Geometry: final body of the model. Coordinates: model frame, mm. Face numbers are marked on the shaded views. A direction names the side the tool comes from. Give positions to 0.01 mm unless a question says otherwise; leave off trailing zeros. Write each loop counter-clockwise with the first axis right and the second up, starting at its lowest first coordinate (ties: lowest second). Pieces come first, ordered by that corner, then holes. Notation, with made-up numbers: (70.25, 77.5) - (111.25, 77.5) arc R35 ccw to (111.25, 110.5) - close; hole circle Ø10 at (-20.75, 17). An arc over 180 degrees is marked (long way). Use CSV: the item, a comma, the result in double quotes. Start each with the question number.
(1) Reachability of the marked faces 1 and 2 from +Z, -Z, +X, -X, +Y, -Y: full face, straight path, thin tool, end or side. Return the list, or none.
(2) Section B-B on x = 0. Output: boundary loops of the cut face in (y, z).
(3) Section D-D on x = -11. Output: boundary loops of the cut face in (y, z), and give its area (3 significant figures).
(4) First-contact query: pin 1 Ø3 at (x, z) = (-3.5, -2) entering from +Y; pin 2 Ø4 at (x, z) = (-4.5, -0.5) entering from -Y; pin 3 Ø1 at (x, y) = (5, 6) entering from +Z; pin 4 Ø4 at (y, z) = (11.5, -6) entering from -X. Flat tips, straight axial feed; report the tip coordinate or a pass-through.
(5) Draft query along X for the marked faces 3, 4 and 5. Return one class per face: released by +X, released by -X, zero draft, split by the parting line, or undercut.
(6) Line query: probe 1 along Y at (x, z) = (0, -4); probe 2 along Y at (x, z) = (0, 1.5); probe 3 along Z at (x, y) = (3.5, 13). Output: solid intervals per line, ascending. Write a range as [from, to].
(7) Section A-A on y = 1.5. Output: boundary loops of the cut face in (x, z), and give its area (3 significant figures).
(8) Section C-C on z = -11.25. Output: boundary loops of the cut face in (x, y).
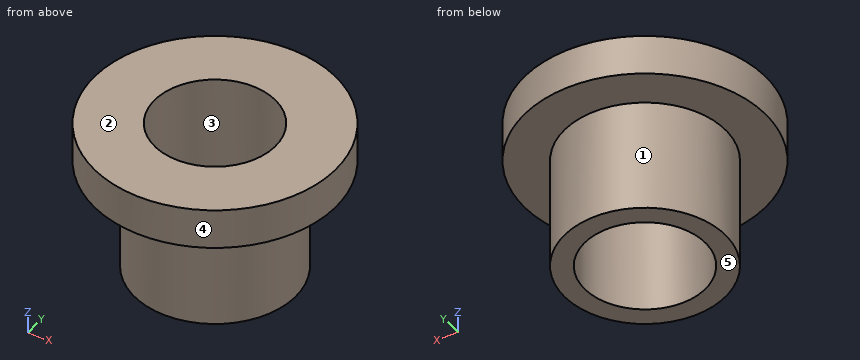
Autodesk Inventor part; units mm, degrees
ref_plane "Work Plane1" through (-46.5047, -36.7959, -17) normal (0, 0, -1) x (0, 1, 0)
ref_plane "Work Plane2" through (-46.5047, -36.7959, -14) normal (0, 0, -1) x (0, 1, 0)
ref_plane "YZ Plane" through (0, 0, 0) normal (1, 0, 0) x (0, 1, 0)
sketch "Sketch1" plane through (0, 0, 0) normal (0, 0, 1) x (1, 0, 0)
  circle A0 centre (0, 1.5) radius 10
  circle A1 centre (0, 1.5) radius 10
  circle A2 centre (0, 1.5) radius 15
  circle A3 centre (0, 1.5) radius 7.5
  point P0 (0, 0)
  dimension "d0" = 30
  dimension "d1" = 15
ref_plane "Work Plane1" through (-46.5047, -36.7959, -17) normal (0, 0, -1) x (0, 1, 0)
ref_plane "Work Plane2" through (-46.5047, -36.7959, -14) normal (0, 0, -1) x (0, 1, 0)
extrude "Extrusion1" add sketch "Sketch1" against normal up to surface (14 mm away) contours A0
sketch "Sketch2" plane through (0, 1.5, 0) normal (0, 0, 1) x (1, 0, 0)
  circle A0 centre (0, 0) radius 10
  circle A1 centre (0, 0) radius 7.5
  circle A2 centre (0, 0) radius 15
  point P0 (0, -1.5)
  dimension "d4" = 30
extrude "Extrusion2" add sketch "Sketch2" along normal blind 5 contours A0 | A2
properties part number "glide lejre bushing" material "Brass, Soft Yellow"
Check values:
1,face 1,"-Z"
1,face 2,"+Z, +X, -X, +Y, -Y"
2,outline,"(-13.5, 0) - (-8.5, 0) - (-8.5, -14) - (-6, -14) - (-6, 5) - (-13.5, 5) - close; (9, -14) - (11.5, -14) - (11.5, 0) - (16.5, 0) - (16.5, 5) - (9, 5) - close"
3,outline,"(-8.7, 0) - (11.7, 0) - (11.7, 5) - (-8.7, 5) - close"
3,area,"102 mm²"
4,pin 1,"stops at y = 11.3"
4,pin 2,"stops at y = -13.28"
4,pin 3,"passes through"
4,pin 4,"stops at x = -6"
5,face 3,"undercut"
5,face 4,"split by the parting line"
5,face 5,"zero draft"
6,probe 1,"y = [-8.5, -6], [9, 11.5]"
6,probe 2,"y = [-13.5, -6], [9, 16.5]"
6,probe 3,"z = [0, 5]"
7,outline,"(-15, 0) - (-10, 0) - (-10, -14) - (-7.5, -14) - (-7.5, 5) - (-15, 5) - close; (7.5, -14) - (10, -14) - (10, 0) - (15, 0) - (15, 5) - (7.5, 5) - close"
7,area,"145 mm²"
8,outline,"circle Ø20 at (0, 1.5); hole circle Ø15 at (0, 1.5)"
